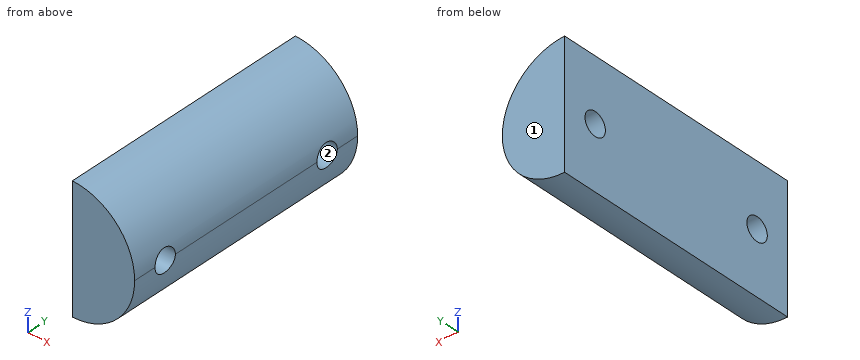
```python
from build123d import *

# Parameters (mm, degrees)
BOSS_EXTRUDE2_DEPTH = 131.3737
SKETCH2_R           = 6
CUT_EXTRUDE1_DEPTH  = 59


with BuildPart() as part:
    # Sketch1 → Boss-Extrude2 (new body)
    with BuildSketch(Plane(origin=(0, 0, 0), x_dir=(1, 0, 0), z_dir=(0, 1, 0))):
        with BuildLine():
            ThreePointArc((32.5, 0), (22.980970389, 22.980970389), (0, 32.5))
            Line((0, 32.5), (0, -32.5))
            ThreePointArc((0, -32.5), (22.980970389, -22.980970389), (32.5, 0))
        make_face()
    extrude(amount=-BOSS_EXTRUDE2_DEPTH)

    # Sketch2 → Cut-Extrude1 (cut)
    with BuildSketch(Plane.ZY):
        with Locations((0, -18)):
            Circle(SKETCH2_R)
        with Locations((0, -113.3737)):
            Circle(SKETCH2_R)
    extrude(amount=-CUT_EXTRUDE1_DEPTH, mode=Mode.SUBTRACT)


solid = part.part
```
Verification items for the finished model (mm, model axes). Face numbers are marked on the shaded views. Round coordinates to 2 decimals unless told otherwise and drop trailing zeros. Order: outer loops, then holes, each group sorted by start corner. A loop starts at its lowest first (then second) coordinate and runs counter-clockwise, first axis right, second up.
1) Cross-section at B-B, the plane y = -14. Record the cut outline in (x, z).
Geometry says:
outline: (0, -32.5) arc R32.5 ccw to (32.19, -4.47) - (0, -4.47) - close; (0, 4.47) - (32.19, 4.47) arc R32.5 ccw to (0, 32.5) - close
2) Depth check by flat-ended pin: pin 1 (12 mm diameter, centred on y = -24.5, z = -11, fed in from +X); pin 2 (3 mm diameter, centred on x = 11, y = -15, fed in from +Z); pin 3 (12 mm diameter, centred on x = 12.5, y = -101.5, fed in from +Z). Enter the tip coordinate at first touch or a pass-through.
Geometry says:
pin 1: stops at x = 32.11
pin 2: stops at z = 31.08
pin 3: stops at z = 31.84
3) Cross-section at D-D, the plane z = -28. Record the cut outline in (x, y).
Geometry says:
outline: (0, -131.37) - (16.5, -131.37) - (16.5, 0) - (0, 0) - close
4) Cross-section at A-A, the plane z = 4. Record the cut outline in (x, y), plus the area to 3 significant figures.
Geometry says:
outline: (0, -131.37) - (32.25, -131.37) - (32.25, -117.85) - (0, -117.85) - close; (0, -108.9) - (32.25, -108.9) - (32.25, -22.47) - (0, -22.47) - close; (0, -13.53) - (32.25, -13.53) - (32.25, 0) - (0, 0) - close
area: 3,660 mm2
5) Material ranges on line 1 (Y direction, x = 10, z = 0); line 2 (Y direction, x = 28.5, z = -1.5); line 3 (Z direction, x = 13, y = -111.5), recorded low to high.
Geometry says:
line 1: y = -131.37 to -119.37, -107.37 to -24, -12 to 0
line 2: y = -131.37 to -119.18, -107.56 to -23.81, -12.19 to 0
line 3: z = -29.79 to -5.7, 5.7 to 29.79
6) Draft check along Z on the marked faces 1 and 2. Enter one of: +Z half, -Z half, draft (parallel to the pull), parting line (faces both ways), or undercut.
Geometry says:
face 1: draft
face 2: undercut
7) Cross-section at C-C, the plane x = 6. Record the cut outline in (y, z), plus the area to 3 significant figures.
Geometry says:
outline: (-131.37, -31.94) - (0, -31.94) - (0, 31.94) - (-131.37, 31.94) - close; hole circle Ø12 at (-113.37, 0); hole circle Ø12 at (-18, 0)
area: 8,170 mm2
